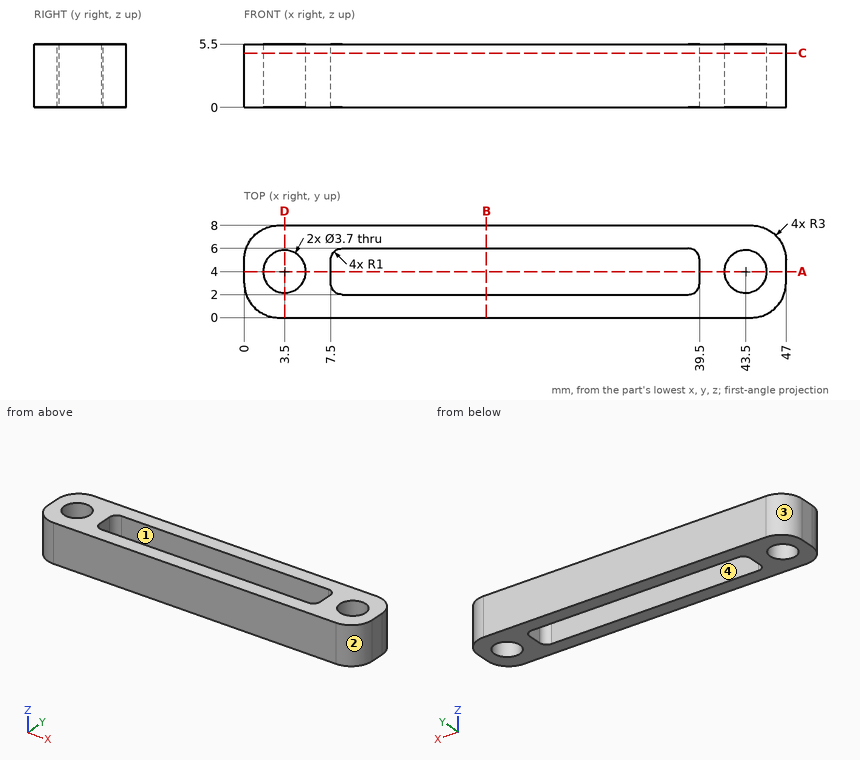
Answer from the drawing. Dimensions are ordinates in mm from the lowest x, y and z of the part. Give positions to 0.01 mm unless a question says otherwise; leave off trailing zeros. Write each loop counter-clockwise with the first axis right and the second up, starting at its lowest first coordinate (ties: lowest second). Pieces come first, ordered by that corner, then holes. Notation, with made-up numbers: (-22.75, -25.5) -> (-12.75, -25.5) arc R30 cw to (-12.75, 4.5) -> close; hole circle Ø3 at (88.5, -8). An arc over 180 degrees is marked (long way). One line per question, with ' | ' between items. Start each with the question number.
1. Section B-B (x = 21) is taken. Determine the outline of the cut face in (y, z), plus the area to 3 significant figures.
2. Section A-A (y = 4) is taken. Determine the outline of the cut face in (x, z).
3. Section C-C (z = 4.7) is taken. Determine the outline of the cut face in (x, y), plus the area to 3 significant figures.
4. Find the intervals of material crossed by probe 1 along Y at (x, z) = (29, 0.25); probe 2 along Y at (x, z) = (3.5, 2.1); probe 3 along X at (y, z) = (5.5, 3.4), in increasing order.
5. Section D-D (x = 3.5) is taken. Determine the outline of the cut face in (y, z), plus the area to 4 significant figures.
6. For a pull along X with two mould halves and no side action, classify the marked faces 1, 2, 3 and 4 as pulls with the +X half, pulls with the -X half, needs draft (parallel to the pull), parting line crosses it, or undercut.
Response values:
1) outline: (0, 0) -> (2, 0) -> (2, 5.5) -> (0, 5.5) -> close; (6, 0) -> (8, 0) -> (8, 5.5) -> (6, 5.5) -> close | area: 22.0 mm2
2) outline: (0, 0) -> (1.65, 0) -> (1.65, 5.5) -> (0, 5.5) -> close; (5.35, 0) -> (7.5, 0) -> (7.5, 5.5) -> (5.35, 5.5) -> close; (39.5, 0) -> (41.65, 0) -> (41.65, 5.5) -> (39.5, 5.5) -> close; (45.35, 0) -> (47, 0) -> (47, 5.5) -> (45.35, 5.5) -> close
3) outline: (0, 3) arc R3 ccw to (3, 0) -> (44, 0) arc R3 ccw to (47, 3) -> (47, 5) arc R3 ccw to (44, 8) -> (3, 8) arc R3 ccw to (0, 5) -> close; hole circle Ø3.7 at (3.5, 4); hole (7.5, 3) arc R1 ccw to (8.5, 2) -> (38.5, 2) arc R1 ccw to (39.5, 3) -> (39.5, 5) arc R1 ccw to (38.5, 6) -> (8.5, 6) arc R1 ccw to (7.5, 5) -> close; hole circle Ø3.7 at (43.5, 4) | area: 220 mm2
4) probe 1: 0 to 2, 6 to 8 | probe 2: 0 to 2.15, 5.85 to 8 | probe 3: 0.04 to 2.42, 4.58 to 7.63, 39.37 to 42.42, 44.58 to 46.96
5) outline: (0, 0) -> (2.15, 0) -> (2.15, 5.5) -> (0, 5.5) -> close; (5.85, 0) -> (8, 0) -> (8, 5.5) -> (5.85, 5.5) -> close | area: 23.65 mm2
6) face 1: undercut | face 2: pulls with the +X half | face 3: pulls with the -X half | face 4: undercut
